Autodesk Inventor part; units mm, degrees
ref_plane "YZ Plane" through (0, 0, 0) normal (1, 0, 0) x (0, 1, 0)
ref_plane "XZ Plane" through (0, 0, 0) normal (0, 1, 0) x (-1, 0, 0)
ref_plane "XY Plane" through (0, 0, 0) normal (0, 0, 1) x (1, 0, 0)
sketch "Sketch1" plane through (0, 0, 0) normal (0, 1, 0) x (-1, 0, 0)
  line L0 (20, 45) -> (-20, 45)
  line L1 (-20, 45) -> (-20, -45)
  line L2 (-20, -45) -> (20, -45)
  line L3 (20, -45) -> (20, 45)
  line L4 (20, 45) -> (-20, -45) construction
  line L5 (-20, 45) -> (20, -45) construction
  arc A0 (-20, -45) -> (20, -45) centre (0, -45) ccw
  line L6 (20, -45) -> (52, -45)
  line L7 (52, -45) -> (52, 45)
  line L8 (52, 45) -> (20, 45)
  line L9 (20, 45) -> (20, -45)
  point P0 (0, 0)
  dimension "d0" = 40
  dimension "d1" = 90
  dimension "d7" = 32
  dimension "d8" = 90
extrude "Extrusion1" add sketch "Sketch1" along normal blind 3.6
sketch "Sketch3" plane through (0, 3.6, 0) normal (0, 1, 0) x (1, 0, 0)
  arc A0 (20, 45) -> (-20, 45) centre (0, 45) ccw
  circle A1 centre (0, 45) radius 20
  circle A2 centre (0, 45) radius 22.5
  point P0 (0, 0)
  point P1 (-19.7203, 38.3333)
  dimension "d13" = 45
extrude "Extrusion3" cut sketch "Sketch3" against normal blind 10 contours A1 A0 | A2
fillet "Fillet2" radius 4 5 edges at (-52, 1.8, -45) (-52, 1.8, 45) (20, 1.8, 45) (-22.5, 1.8, -45) (20, 1.8, -34.6922)
sketch "Sketch4" plane through (0, 3.6, 0) normal (0, 1, 0) x (1, 0, 0)
  circle A0 centre (-5, -20) radius 22.5
  line L0 (20, -41) -> (20, 23.8754)
  line L1 (-48, -45) -> (16, -45)
  point P0 (0, 0)
  dimension "d14" = 45
  dimension "d15" = 25
  dimension "d16" = 25
extrude "Extrusion4" cut sketch "Sketch4" against normal blind 10
sketch "Sketch5" plane through (0, 0, 0) normal (0, -1, 0) x (1, 0, 0)
  circle A0 centre (-27.5, -40.5) radius 1.625
  circle A1 centre (15.5, 40.5) radius 1.625
  circle A2 centre (15.5, -19.5) radius 1.625
  line L0 (20, 41) -> (20, -23.8754)
  line L1 (-48, 45) -> (16, 45)
  line L2 (-26.1964, -45) -> (-48, -45)
  line L3 (-52, -41) -> (-52, 41)
  point P0 (0, 0)
  dimension "d19" = 3.25
  dimension "d21" = 3.25
  dimension "d22" = 3.25
  dimension "d23" = 4.5
  dimension "d24" = 4.5
  dimension "d25" = 4.5
  dimension "d26" = 56.75
  dimension "d27" = 4.5
  dimension "d28" = 24.5
extrude "Extrusion5" cut sketch "Sketch5" against normal blind 10
sketch "Sketch6" plane through (0, 3.6, 0) normal (0, 1, 0) x (1, 0, 0)
  circle A0 centre (-48, -40) radius 1.575
  line L0 (-48, -45) -> (16, -45)
  line L1 (-52, 41) -> (-52, -41)
  point P0 (0, 0)
  dimension "d31" = 3.15
  dimension "d32" = 5
  dimension "d33" = 4
extrude "Extrusion6" cut sketch "Sketch6" against normal blind 10
properties part number "p1"
The model under review builds one solid part; all positions refer to its coordinate system, in mm. Round coordinates to 2 decimals unless told otherwise and drop trailing zeros. Order: outer loops, then holes, each group sorted by start corner. A loop starts at its lowest first (then second) coordinate and runs counter-clockwise, first axis right, second up. Notation, with made-up numbers: (65.5, -33.5) - (99.5, -33.5) arc R11 ccw to (99.5, -23.5) - close; hole circle Ø1 at (35, 81.25). An arc over 180 degrees is marked (long way). Use one line per item in the form item = value.
Q1. Clearance check with a flat-ended pin moving along its axis: P1, Ø3.5, axis at x = -48, z = 40, coming from the -Y side. State where the tip first meets the part, or that it passes through.
Response values:
P1 = 0
Q2. To check wall thickness, follow line 1 (Z direction, x = 15.5, y = 1.25) (3 decimals); line 2 (Z direction, x = -48, y = 1.3) (3 decimals); line 3 (X direction, y = 0.45, z = 40) (3 decimals). State the ranges of each line that lie inside material, in increasing order.
Response values:
line_1 = -27.844 to -21.125, -17.875 to 10.726, 29.274 to 38.875, 42.125 to 45
line_2 = -45 to 38.425, 41.575 to 45
line_3 = -52 to -49.575, -46.425 to -15.308, 5.308 to 13.954, 17.046 to 20
Q3. Add section A-A on z = -19.5. Give the boundary of the cut face in (x, y) (3 decimals), then the cut area to 4 significant figures.
Response values:
outline = (-52, 0) - (13.875, 0) - (13.875, 3.6) - (-52, 3.6) - close; (17.125, 0) - (20, 0) - (20, 3.6) - (17.125, 3.6) - close
area = 247.5 mm^2
Q4. Add section B-B on x = -5. Give the boundary of the cut face in (y, z), then the cut area to 3 significant figures.
Response values:
outline = (0, -23.06) - (3.6, -23.06) - (3.6, -2.5) - (0, -2.5) - close; (0, 42.5) - (3.6, 42.5) - (3.6, 45) - (0, 45) - close
area = 83.0 mm^2
Q5. Add section C-C on y = 1.1. Give the boundary of the cut face in (x, z) (3 decimals), then the cut area to 3 significant figures.
Response values:
outline = (-52, -41) arc R4 ccw to (-48, -45) - (-26.196, -45) arc R4 ccw to (-22.242, -41.604) arc R22.5 cw to (13.585, -27.064) arc R4 ccw to (20, -23.875) - (20, 41) arc R4 ccw to (16, 45) - (-48, 45) arc R4 ccw to (-52, 41) - close; hole circle Ø3.15 at (-48, 40); hole circle Ø3.25 at (-27.5, -40.5); hole circle Ø45 at (-5, 20); hole circle Ø3.25 at (15.5, -19.5); hole circle Ø3.25 at (15.5, 40.5)
area = 4,050 mm^2
Q6. Mouldability with a two-part tool opening along X and no side actions: class faces 1 (the cylindrical face through (-49.573, 1.825, 39.931)), 2 (the flat face through (20, 2, 9)), 3 (the flat face through (-52, 2, -1)), 4 (the flat face through (-23, 0, 1)) as pulls with the +X half, pulls with the -X half, needs draft (parallel to the pull), parting line crosses it, or undercut.
Response values:
face_1 = undercut
face_2 = pulls with the +X half
face_3 = pulls with the -X half
face_4 = needs draft
